Autodesk Inventor part; units mm, degrees
ref_plane "YZ Plane" through (0, 0, 0) normal (1, 0, 0) x (0, 1, 0)
ref_plane "XZ Plane" through (0, 0, 0) normal (0, 1, 0) x (-1, 0, 0)
ref_plane "XY Plane" through (0, 0, 0) normal (0, 0, 1) x (1, 0, 0)
sketch "Sketch1" plane through (0, 0, 0) normal (0, 1, 0) x (-1, 0, 0)
  circle A0 centre (0, 0) radius 46.5
  circle A1 centre (0, 0) radius 47.5
  dimension "d0" = 93
  dimension "d1" = 95
extrude "Extrusion1" add sketch "Sketch1" along normal blind 85
sketch "Sketch2" plane through (0, 0, 0) normal (0, -1, 0) x (1, 0, 0)
  circle A0 centre (0, 0) radius 41.5
  circle A1 centre (0, 0) radius 47.5
  dimension "d4" = 83
extrude "Extrusion2" add sketch "Sketch2" against normal blind 2
sketch "Sketch3" plane through (0, 0, 0) normal (0, -1, 0) x (1, 0, 0)
  circle A0 centre (0, 44.5) radius 1.5
  circle A1 centre (-38.5381, 22.25) radius 1.5
  circle A2 centre (-38.5381, -22.25) radius 1.5
  circle A3 centre (0, -44.5) radius 1.5
  circle A4 centre (38.5381, -22.25) radius 1.5
  circle A5 centre (38.5381, 22.25) radius 1.5
  point P0 (0, 0)
  dimension "d7" = 3
  dimension "d8" = 44.5
  dimension "d11" = 360
extrude "Extrusion3" cut sketch "Sketch3" against normal blind 10 contours A1 | A2 | A4 | A5
properties part number "Outer casing"
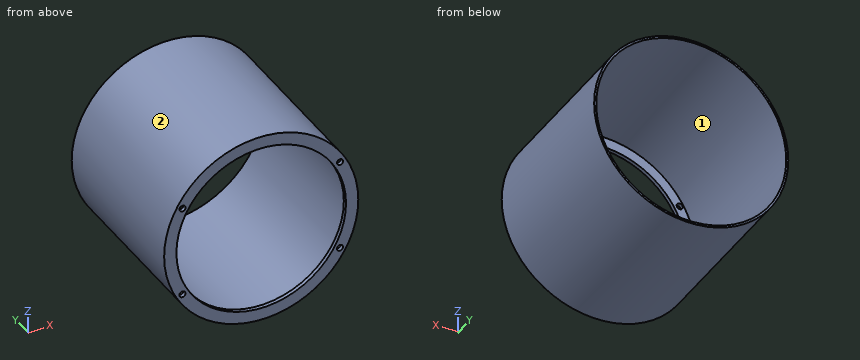
Read the model definition and answer for the solid it produces. Units are mm, in the model's axes. Face numbers are marked on the shaded views. Coordinates: 2 decimals unless noted, no trailing zeros. Order: outer loops, then holes, each group sorted by start corner. A loop starts at its lowest first (then second) coordinate and runs counter-clockwise, first axis right, second up. Notation, with made-up numbers: (-2.5, 76.25) - (16.5, 76.25) arc R17 cw to (16.5, 105.25) - close; hole circle Ø7 at (48, 83.25). An arc over 180 degrees is marked (long way). Answer as a JSON object with one key per item and string values. Group by question number.
Item 1: Section A-A (z = 0) is taken. Give the vertices of the cut face in (x, y).
Item 2: Section D-D (y = 53) is taken. Give the vertices of the cut face in (x, z).
Item 3: Flat-ended cylindrical pins translate along their axes: P1, Ø1.8, axis at x = -38.54, z = 22.25, coming from the -Y side; P2, Ø3.5, axis at x = 38.54, z = 22.25, coming from the +Y side; P3, Ø1.5, axis at x = -35, y = 63, coming from the +Z side; P4, Ø5, axis at x = 25.5, y = 16.5, coming from the +Z side. Find the tip coordinate at first contact, or state that the pin passes through.
Item 4: Consider probe 1 along Z at (x, y) = (-28.5, 12); probe 2 along Z at (x, y) = (-22, 33.5); probe 3 along X at (y, z) = (70.5, 29.5). Determine where each line is inside the solid, lowest interval first. Write a range as from..to.
Item 5: Section B-B (x = 0) is taken. Give the vertices of the cut face in (y, z), plus the area to 3 significant figures.
Item 6: Section C-C (z = -22.25) is taken. Give the vertices of the cut face in (x, y).
Item 7: The mould has two halves that part along Z. Classify the marked faces 1 and 2: +Z half, -Z half, draft (parallel to the pull), parting line (faces both ways), or undercut.
Results are:
{
 "1": {"outline": "(-47.5, 0) - (-41.5, 0) - (-41.5, 2) - (-46.5, 2) - (-46.5, 85) - (-47.5, 85) - close; (41.5, 0) - (47.5, 0) - (47.5, 85) - (46.5, 85) - (46.5, 2) - (41.5, 2) - close"},
 "2": {"outline": "circle Ø95 at (0, 0); hole circle Ø93 at (0, 0)"},
 "3": {"P1": "passes through", "P2": "stops at y = 2", "P3": "stops at z = 32.91", "P4": "stops at z = 41.56"},
 "4": {"probe 1": "z = -38..-36.74, 36.74..38", "probe 2": "z = -42.1..-40.97, 40.97..42.1", "probe 3": "x = -37.23..-35.94, 35.94..37.23"},
 "5": {"outline": "(0, -47.5) - (85, -47.5) - (85, -46.5) - (2, -46.5) - (2, -41.5) - (0, -41.5) - close; (0, 41.5) - (2, 41.5) - (2, 46.5) - (85, 46.5) - (85, 47.5) - (0, 47.5) - close", "area": "190 mm^2"},
 "6": {"outline": "(-41.97, 0) - (-40.04, 0) - (-40.04, 2) - (-40.83, 2) - (-40.83, 85) - (-41.97, 85) - close; (-37.04, 0) - (-35.03, 0) - (-35.03, 2) - (-37.04, 2) - close; (35.03, 0) - (37.04, 0) - (37.04, 2) - (35.03, 2) - close; (40.04, 0) - (41.97, 0) - (41.97, 85) - (40.83, 85) - (40.83, 2) - (40.04, 2) - close"},
 "7": {"face 1": "undercut", "face 2": "parting line"}
}
